Could you check a few things on this drawing? It's one solid part, dimensions in mm from its lowest x, y, z. Give positions to 0.01 mm unless a question says otherwise; leave off trailing zeros. Order: outer loops, then holes, each group sorted by start corner. A loop starts at its lowest first (then second) coordinate and runs counter-clockwise, first axis right, second up.
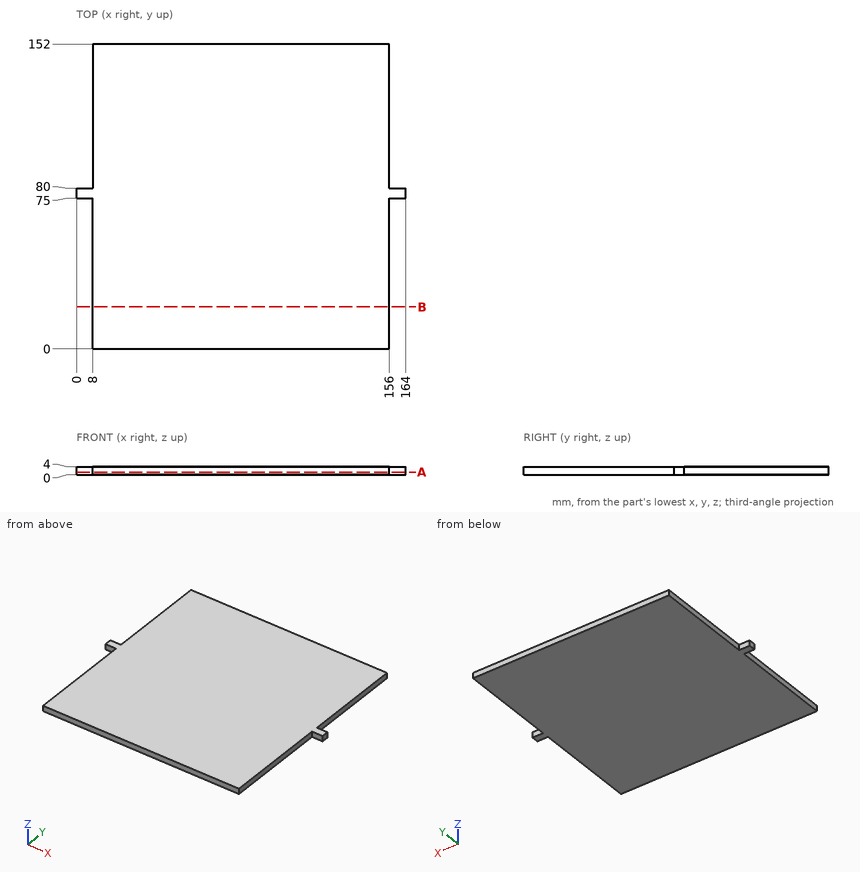
Q1. If we section it at A-A on z = 1.45: List the corners of the cut face in (x, y) for me.
Filled sheet:
outline: (0, 75) - (8, 75) - (8, 0) - (156, 0) - (156, 75) - (164, 75) - (164, 80) - (156, 80) - (156, 152) - (8, 152) - (8, 80) - (0, 80) - close
Q2. I'm going to push flat-ended pins straight in: P1, Ø4, axis at x = 143.5, y = 68, coming from the -Z side; P2, Ø1.2, axis at y = 35, z = 2.5, coming from the +X side; P3, Ø1.2, axis at x = 4, z = 1.5, coming from the -Y side; P4, Ø1.2, axis at x = 4.5, z = 1.5, coming from the +Y side. Where does each tip first touch, or does it pass through?
Filled sheet:
P1: stops at z = 0
P2: stops at x = 156
P3: stops at y = 75
P4: stops at y = 80
Q3. If we section it at B-B on y = 21: List the corners of the cut face in (x, z) for me.
Filled sheet:
outline: (8, 0) - (156, 0) - (156, 4) - (8, 4) - close
Q4. I need wall thicknesses on L1, parallel to X at y = 47.5, z = 3.85; L2, parallel to Y at x = 7, z = 2.9. Which ranges of each line are inside material? Lowest first, please.
Filled sheet:
L1: x = 8 to 156
L2: y = 75 to 80
